The listing builds one solid part. Answer for the finished solid, in the listing's coordinates (mm). Coordinates: 2 decimals unless noted, no trailing zeros. Write each loop counter-clockwise with the first axis right and the second up, starting at its lowest first coordinate (ties: lowest second). Pieces come first, ordered by that corner, then holes.
(1) For a pull along X with two mould halves and no side action, classify faces 1 (the flat face through (12, 2, 0)), 2 (the flat face through (25, 2, -148)), 3 (the cylindrical face through (12.6, 2.5, -103)) as +X half, -X half, draft (parallel to the pull), parting line (faces both ways), or undercut.
(2) The part is cut by section B-B on z = -12.5. Determine the outline of the cut face in (x, y), plus the area to 3 significant figures.
(3) The part is cut by section A-A on z = -266. Determine the outline of the cut face in (x, y).
(4) Straight lines are drawn through the part: line 1 (X direction, y = 3.65, z = -100); line 2 (Z direction, x = 10.75, y = 1.9); line 3 (Z direction, x = 11.5, y = 1.4). For each, find the intervals that lie inside material, in ascending order.
from build123d import *

# Parameters (mm, degrees)
SKETCH1_W           = 25
SKETCH1_H           = 300
SKETCH1_R           = 3
BOSS_EXTRUDE1_DEPTH = 5
SKETCH2_R           = 4
CUT_EXTRUDE1_DEPTH  = 302.081384346


with BuildPart() as part:
    # Sketch1 → Boss-Extrude1 (new body)
    with BuildSketch(Plane(origin=(0, 0, 0), x_dir=(1, 0, 0), z_dir=(0, 1, 0))):
        with Locations((12.5, 150)):
            Rectangle(SKETCH1_W, SKETCH1_H)
        with Locations(Location((12.5, 12.5, 0), (0, 0, 270))):
            Circle(SKETCH1_R, mode=Mode.SUBTRACT)
        with Locations(Location((12.5, 100, 0), (0, 0, 270))):
            Circle(SKETCH1_R, mode=Mode.SUBTRACT)
    extrude(amount=BOSS_EXTRUDE1_DEPTH)

    # Sketch2 → Cut-Extrude1 (cut, through all)
    with BuildSketch(Plane(origin=(0, 5, 0), x_dir=(1, 0, 0), z_dir=(0, 1, 0))):
        with Locations(Location((12.3, 266, 0), (0, 0, 270))):
            Circle(SKETCH2_R)
    extrude(amount=-CUT_EXTRUDE1_DEPTH, mode=Mode.SUBTRACT)


solid = part.part
Model answer:
1. face 1: draft
1. face 2: +X half
1. face 3: undercut
2. outline: (0, 0) - (9.5, 0) - (9.5, 5) - (0, 5) - close; (15.5, 0) - (25, 0) - (25, 5) - (15.5, 5) - close
2. area: 95.0 mm2
3. outline: (0, 0) - (8.3, 0) - (8.3, 5) - (0, 5) - close; (16.3, 0) - (25, 0) - (25, 5) - (16.3, 5) - close
4. line 1: x = 0 to 9.5, 15.5 to 25
4. line 2: z = -300 to -269.69, -262.31 to -102.44, -97.56 to -14.94, -10.06 to 0
4. line 3: z = -300 to -269.92, -262.08 to -102.83, -97.17 to -15.33, -9.67 to 0
